```python
from build123d import *

# Parameters (mm, degrees)
F0_R     = 55
F1_DEPTH = 3


with BuildPart() as f1:
    # F0 (on Top) → F1 (new body)
    with BuildSketch(Plane.XY):
        with BuildLine():
            Line((60, 1.5), (64.98269, 1.5))
            ThreePointArc((64.98269, 1.5), (63.751043, 12.680871), (60.610202, 23.48198))
            Line((60.610202, 23.48198), (56.006797, 21.575187))
            Line((56.006797, 21.575187), (54.858747, 24.346825))
            Line((54.858747, 24.346825), (59.462152, 26.253618))
            ThreePointArc((59.462152, 26.253618), (54.045525, 36.112065), (47.010361, 44.889041))
            Line((47.010361, 44.889041), (43.487067, 41.365747))
            Line((43.487067, 41.365747), (41.365747, 43.487067))
            Line((41.365747, 43.487067), (44.889041, 47.010361))
            ThreePointArc((44.889041, 47.010361), (36.112065, 54.045525), (26.253618, 59.462152))
            Line((26.253618, 59.462152), (24.346825, 54.858747))
            Line((24.346825, 54.858747), (21.575187, 56.006797))
            Line((21.575187, 56.006797), (23.48198, 60.610202))
            ThreePointArc((23.48198, 60.610202), (12.680871, 63.751043), (1.5, 64.98269))
            Line((1.5, 64.98269), (1.5, 60))
            Line((1.5, 60), (-1.5, 60))
            Line((-1.5, 60), (-1.5, 64.98269))
            ThreePointArc((-1.5, 64.98269), (-12.680871, 63.751043), (-23.48198, 60.610202))
            Line((-23.48198, 60.610202), (-21.575187, 56.006797))
            Line((-21.575187, 56.006797), (-24.346825, 54.858747))
            Line((-24.346825, 54.858747), (-26.253618, 59.462152))
            ThreePointArc((-26.253618, 59.462152), (-36.112065, 54.045525), (-44.889041, 47.010361))
            Line((-44.889041, 47.010361), (-41.365747, 43.487067))
            Line((-41.365747, 43.487067), (-43.487067, 41.365747))
            Line((-43.487067, 41.365747), (-47.010361, 44.889041))
            ThreePointArc((-47.010361, 44.889041), (-54.045525, 36.112065), (-59.462152, 26.253618))
            Line((-59.462152, 26.253618), (-54.858747, 24.346825))
            Line((-54.858747, 24.346825), (-56.006797, 21.575187))
            Line((-56.006797, 21.575187), (-60.610202, 23.48198))
            ThreePointArc((-60.610202, 23.48198), (-63.751043, 12.680871), (-64.98269, 1.5))
            Line((-64.98269, 1.5), (-60, 1.5))
            Line((-60, 1.5), (-60, -1.5))
            Line((-60, -1.5), (-64.98269, -1.5))
            ThreePointArc((-64.98269, -1.5), (-63.751043, -12.680871), (-60.610202, -23.48198))
            Line((-60.610202, -23.48198), (-56.006797, -21.575187))
            Line((-56.006797, -21.575187), (-54.858747, -24.346825))
            Line((-54.858747, -24.346825), (-59.462152, -26.253618))
            ThreePointArc((-59.462152, -26.253618), (-54.045525, -36.112065), (-47.010361, -44.889041))
            Line((-47.010361, -44.889041), (-43.487067, -41.365747))
            Line((-43.487067, -41.365747), (-41.365747, -43.487067))
            Line((-41.365747, -43.487067), (-44.889041, -47.010361))
            ThreePointArc((-44.889041, -47.010361), (-36.112065, -54.045525), (-26.253618, -59.462152))
            Line((-26.253618, -59.462152), (-24.346825, -54.858747))
            Line((-24.346825, -54.858747), (-21.575187, -56.006797))
            Line((-21.575187, -56.006797), (-23.48198, -60.610202))
            ThreePointArc((-23.48198, -60.610202), (-12.680871, -63.751043), (-1.5, -64.98269))
            Line((-1.5, -64.98269), (-1.5, -60))
            Line((-1.5, -60), (0, -60))
            Line((0, -60), (1.5, -60))
            Line((1.5, -60), (1.5, -64.98269))
            ThreePointArc((1.5, -64.98269), (12.680871, -63.751043), (23.48198, -60.610202))
            Line((23.48198, -60.610202), (21.575187, -56.006797))
            Line((21.575187, -56.006797), (24.346825, -54.858747))
            Line((24.346825, -54.858747), (26.253618, -59.462152))
            ThreePointArc((26.253618, -59.462152), (36.112065, -54.045525), (44.889041, -47.010361))
            Line((44.889041, -47.010361), (41.365747, -43.487067))
            Line((41.365747, -43.487067), (43.487067, -41.365747))
            Line((43.487067, -41.365747), (47.010361, -44.889041))
            ThreePointArc((47.010361, -44.889041), (54.045525, -36.112065), (59.462152, -26.253618))
            Line((59.462152, -26.253618), (54.858747, -24.346825))
            Line((54.858747, -24.346825), (56.006797, -21.575187))
            Line((56.006797, -21.575187), (60.610202, -23.48198))
            ThreePointArc((60.610202, -23.48198), (63.751043, -12.680871), (64.98269, -1.5))
            Line((64.98269, -1.5), (60, -1.5))
            Line((60, -1.5), (60, 1.5))
        make_face()
        Circle(F0_R, mode=Mode.SUBTRACT)
    extrude(amount=F1_DEPTH)


solid = f1.part
```
Design review of the part built by this model. Coordinates are the model's own, in mm. A direction names the side the tool comes from. Coordinates: 2 decimals unless noted, no trailing zeros. Write each loop counter-clockwise with the first axis right and the second up, starting at its lowest first coordinate (ties: lowest second). Pieces come first, ordered by that corner, then holes.
1) Add section A-A (y = 0). Write out the cut boundary in (x, z).
2) To check wall thickness, follow L1, parallel to Y at x = 0, z = 0.65; L2, parallel to Y at x = 58.5, z = 2.85; L3, parallel to X at y = -22, z = 1.8. State the ranges of each line that lie inside material, in increasing order.
3) Mouldability with a two-part tool opening along Y and no side actions: class faces 1 (the flat face through (-22.98, -55.425, 1.479)), 2 (the cylindrical face through (-12.53, 63.78, 1.48)), 3 (the flat face through (-1.5, -63, 1)), 4 (the flat face through (25.287, -57.128, 1.479)) as +Y half, -Y half, draft (parallel to the pull), parting line (faces both ways), or undercut.
4) Machinability: for faces 5 (the flat face through (45.27, 43.15, 1.48)), 6 (the flat face through (-57.193, 25.314, 1.479)), 7 (the cylindrical face through (-53.96, 36.24, 1.48)), 8 (the flat face through (0, -60, 1)), which of the approach directions +Z, -Z, +X, -X, +Y, -Y give a long, thin tool a straight path to every point of the face, cutting with its end or side? Answer none if there is none.
5) Insertion check: pin 1 (0.9 mm diameter, centred on x = 0, z = 1, fed in from +Y); pin 2 (0.9 mm diameter, centred on x = -0.5, z = 1.5, fed in from -Y). Each pin has a flat end and moves straight along its axis. Give the tip position at first contact, or say it passes through.
Check result:
1. outline: (-60, 0) - (-55, 0) - (-55, 3) - (-60, 3) - close; (55, 0) - (60, 0) - (60, 3) - (55, 3) - close
2. L1: y = -60 to -55, 55 to 60
2. L2: y = -28.33 to -25.86, -22.61 to 22.61, 25.86 to 28.33
2. L3: x = -61.16 to -57.03, -55.83 to -50.41, 50.41 to 55.83, 57.03 to 61.16
3. face 1: undercut
3. face 2: +Y half
3. face 3: draft
3. face 4: -Y half
4. face 5: +Z, -Z
4. face 6: +Z, -Z, -X
4. face 7: +Z, -Z, -X, +Y
4. face 8: +Z, -Z, -Y
5. pin 1: stops at y = 60
5. pin 2: stops at y = -60
